The listing builds one solid part. Answer for the finished solid, in the listing's coordinates (mm). Face numbers are marked on the shaded views. Coordinates: 2 decimals unless noted, no trailing zeros. Loops run counter-clockwise (first coordinate to the right, second up) from the corner with the lowest first, then second, coordinate; pieces in that order, holes last. Notation, with made-up numbers: M 83,79.25 L 99,79.25 A23 cw 99,112.25 Z; hole C 30.5,59.5 d3. An arc over 180 degrees is marked long. Return JSON: item names as keys, results as strings. Group by question number.
1. Given P1, Ø6, axis at x = 6, y = 4.5, coming from the -Z side, flat-ended and moving along its own axis, determine where the tip first touches the part or whether it passes through.
2. Straight lines are drawn through the part: L1, parallel to Y at x = 6.15, z = 2.15; L2, parallel to X at y = 1.75, z = 2.9; L3, parallel to X at y = 1.25, z = 2.2. For each, find the intervals that lie inside material, in ascending order. Write a range as from..to.
3. Section B-B (x = -5) is taken. Write down the section's boundary in (y, z) (3 decimals).
4. Section D-D (x = 6.15) is taken. Write down the section's boundary in (y, z) (3 decimals), then the cut area to 3 significant figures.
5. Section C-C (z = 1.35) is taken. Count the separate pieces of the cut face and the enclosed holes in it, then the cut area to 3 significant figures.
6. The mould has two halves that part along X. Classify the marked faces 1, 2 and 3: pulls with the +X half, pulls with the -X half, needs draft (parallel to the pull), parting line crosses it, or undercut.
7. Section A-A (y = 0) is taken. Write down the section's boundary in (x, z) (3 decimals), then the cut area to 3 significant figures.
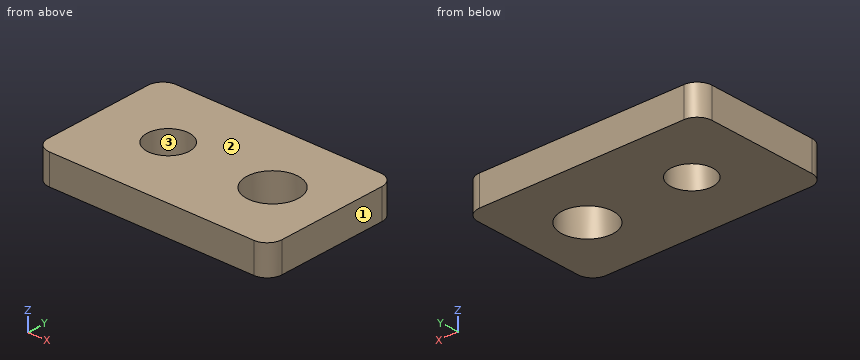
```python
from build123d import *

# Parameters (mm, degrees)
SKETCH1_W            = 25
SKETCH1_H            = 15
SKETCH1_R            = 2.5
BOSS_EXTRUDE1_DEPTH  = 3.175
M5_CLEARANCE_HOLE1_D = 5.5
FILLET1_R            = 1.5875
M4_CLEARANCE_HOLE2_D = 4.5


with BuildPart() as part:
    # Sketch1 → Boss-Extrude1 (new body)
    # profile 1 of 2: a face of its own
    with BuildSketch(Plane.XY):
        Rectangle(SKETCH1_W, SKETCH1_H)
        with Locations((6.15, 0)):
            Circle(SKETCH1_R, mode=Mode.SUBTRACT)
    # profile 2 of 2: a face of its own
    with BuildSketch(Plane.XY):
        with Locations((6.15, 0)):
            Circle(SKETCH1_R)
    extrude(amount=BOSS_EXTRUDE1_DEPTH)

    # M5 Clearance Hole1 (through all)
    with Locations(Plane.XY.offset(3.175)):
        with Locations((6.15, 0)):
            Hole(M5_CLEARANCE_HOLE1_D / 2)

    # Fillet1
    fillet1_edges = [part.edges().sort_by_distance(p)[0] for p in [
        (12.5, -7.5, 1.5875),
        (-12.5, -7.5, 1.5875),
        (-12.5, 7.5, 1.5875),
        (12.5, 7.5, 1.5875),
    ]]
    fillet(fillet1_edges, radius=FILLET1_R)

    # M4 Clearance Hole2 (through all)
    with Locations(Plane.XY.offset(3.175)):
        with Locations((-5, 0)):
            Hole(M4_CLEARANCE_HOLE2_D / 2)


solid = part.part
```
Worked out:
{
 "1": {"P1": "z = 0"},
 "2": {"L1": "-7.5..-2.75, 2.75..7.5", "L2": "-12.5..-6.41, -3.59..4.03, 8.27..12.5", "L3": "-12.5..-6.87, -3.13..3.7, 8.6..12.5"},
 "3": {"outline": "M -7.5,0 L -2.25,0 L -2.25,3.175 L -7.5,3.175 Z; M 2.25,0 L 7.5,0 L 7.5,3.175 L 2.25,3.175 Z"},
 "4": {"outline": "M -7.5,0 L -2.75,0 L -2.75,3.175 L -7.5,3.175 Z; M 2.75,0 L 7.5,0 L 7.5,3.175 L 2.75,3.175 Z", "area": "30.2 mm^2"},
 "5": {"separate pieces": "1", "enclosed holes": "2", "area": "333 mm^2"},
 "6": {"face 1": "pulls with the +X half", "face 2": "needs draft", "face 3": "undercut"},
 "7": {"outline": "M -12.5,0 L -7.25,0 L -7.25,3.175 L -12.5,3.175 Z; M -2.75,0 L 3.4,0 L 3.4,3.175 L -2.75,3.175 Z; M 8.9,0 L 12.5,0 L 12.5,3.175 L 8.9,3.175 Z", "area": "47.6 mm^2"}
}
